Geometry: see drawing. Coordinates: mm, zero at the bounding-box minimum. A direction names the side the tool comes from. Round coordinates to 2 decimals unless told otherwise and drop trailing zeros. Write each loop counter-clockwise with the first axis right and the second up, starting at its lowest first coordinate (ties: lowest second). Pieces come first, ordered by that corner, then holes. Notation, with made-up numbers: M 65,64.5 L 99,64.5 A26 cw 99,88.5 Z; hole C 59,70 d5. An arc over 180 degrees is marked long. Use one line per item in the form item = value. Start each with the question number.
Item 1: Section query A-A (z = 10.5). Return loops of the section in (x, y).
Item 2: Ray query, probe 1 along Y at (x, z) = (36, 31.5); probe 2 along X at (y, z) = (71.5, 34.5); probe 3 along Z at (x, y) = (21, 33.5). Return the intervals inside material, ascending.
Item 3: Reachability of the marked faces 5 and 6 from +Z, -Z, +X, -X, +Y, -Y: full face, straight path, thin tool, end or side. Return the list, or none.
Item 4: Pull-direction query (Y, two-part tool) for the marked faces 1, 2, 3 and 4; classes: pulls with the +Y half, pulls with the -Y half, needs draft (parallel to the pull), parting line crosses it, or undercut.
Item 5: Section query C-C (y = 20). Return loops of the section in (x, z), and give its area (3 significant figures).
Item 6: Section query B-B (x = 78.5). Return loops of the section in (y, z), and give its area (3 significant figures).
Item 7: Pin query (flat end, axial travel): pin 1 Ø6 at (x, y) = (28, 39.5) entering from +Z. Return the tip coordinate at first contact, or that it passes through.
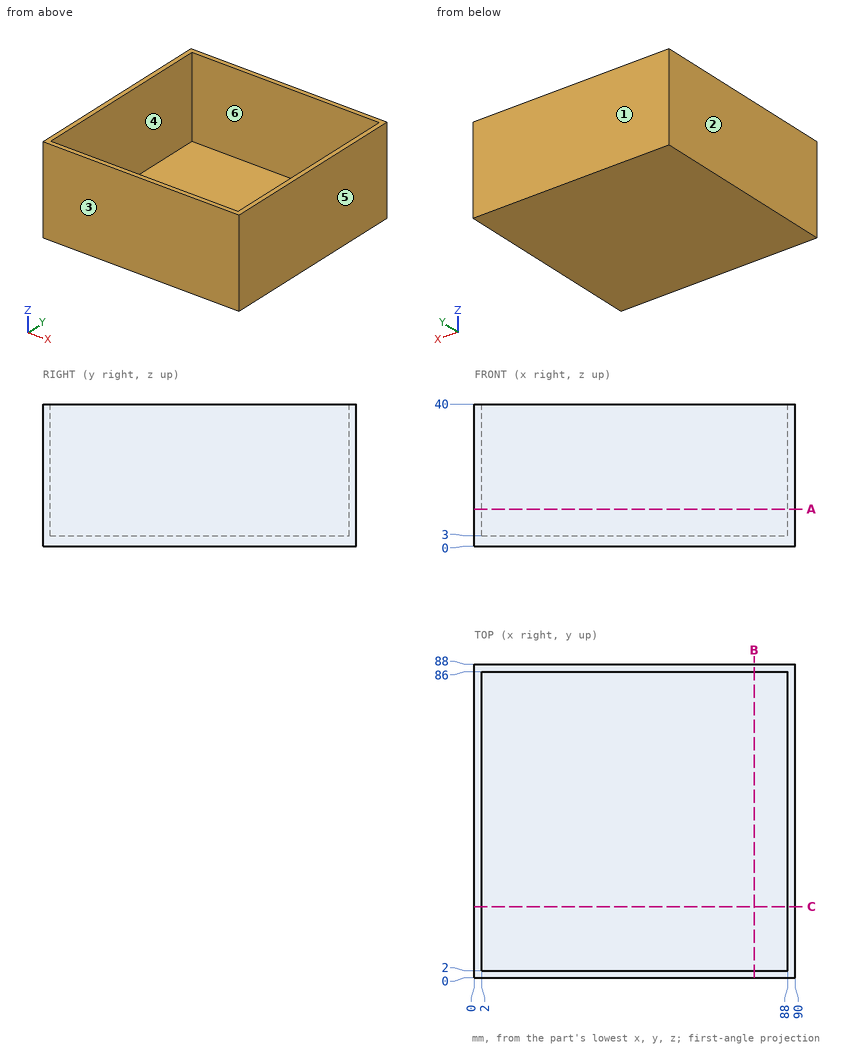
Working result:
q1.outline = M 0,0 L 90,0 L 90,88 L 0,88 Z; hole M 2,2 L 88,2 L 88,86 L 2,86 Z
q2.probe_1 = 0 to 2, 86 to 88
q2.probe_2 = 0 to 2, 88 to 90
q2.probe_3 = 0 to 3
q3.face_5 = +Z, -Z, +X, +Y, -Y
q3.face_6 = +Z
q4.face_1 = pulls with the +Y half
q4.face_2 = needs draft
q4.face_3 = pulls with the -Y half
q4.face_4 = undercut
q5.outline = M 0,0 L 90,0 L 90,40 L 88,40 L 88,3 L 2,3 L 2,40 L 0,40 Z
q5.area = 418 mm²
q6.outline = M 0,0 L 88,0 L 88,40 L 86,40 L 86,3 L 2,3 L 2,40 L 0,40 Z
q6.area = 412 mm²
q7.pin_1 = 3
